Could you check a few things on this drawing? It's one solid part, dimensions in mm from its lowest x, y, z. Coordinates: 2 decimals unless noted, no trailing zeros. Order: outer loops, then holes, each group sorted by start corner. A loop starts at its lowest first (then second) coordinate and runs counter-clockwise, first axis right, second up.
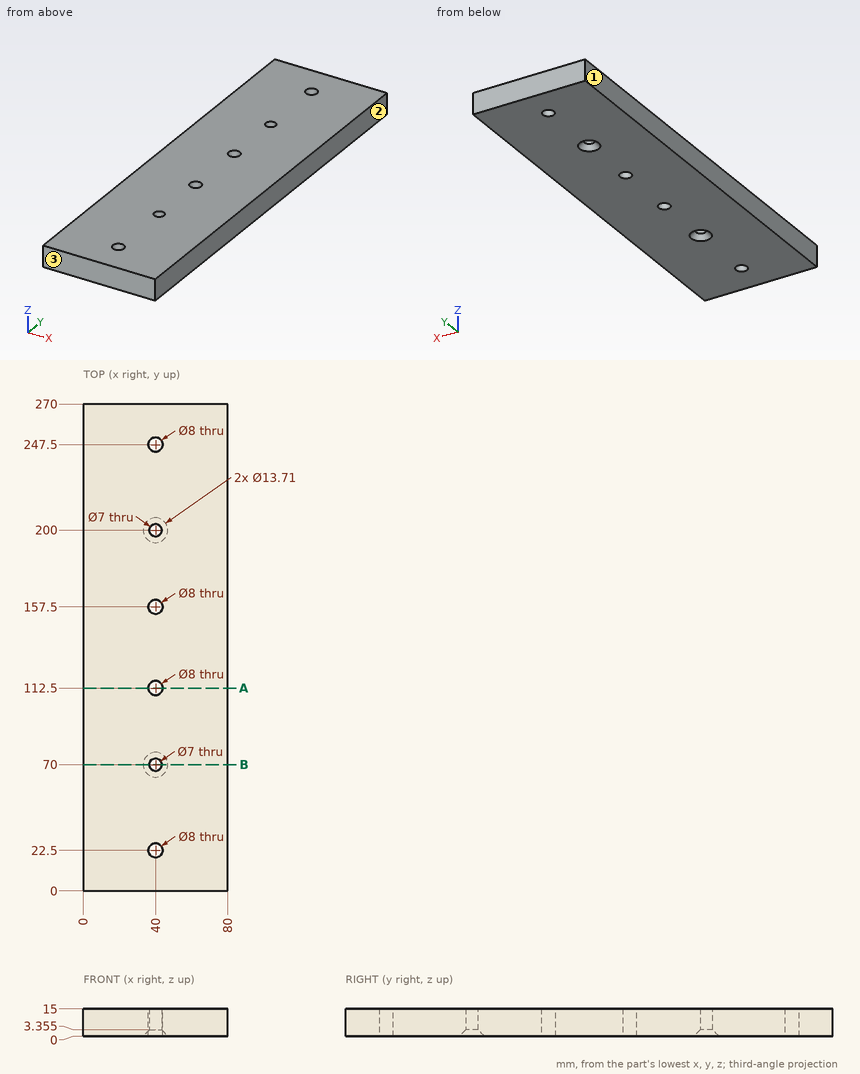
1. Imagine slicing it at A-A on y = 112.5. Please give me the cut outline in (x, z).
Completed:
outline: (0, 0) - (36, 0) - (36, 15) - (0, 15) - close; (44, 0) - (80, 0) - (80, 15) - (44, 15) - close
2. Please list where these lines run through material, in increasing order: probe 1 along X at (y, z) = (70, 10.5); probe 2 along X at (y, z) = (112.5, 4.5).
Completed:
probe 1: x = 0 to 36.5, 43.5 to 80
probe 2: x = 0 to 36, 44 to 80
3. Thinking about a two-plate mould opening in X: for the marked faces 1, 2 and 3, which applies, pulls with the +X half, pulls with the -X half, needs draft (parallel to the pull), parting line crosses it, or undercut?
Completed:
face 1: pulls with the -X half
face 2: pulls with the +X half
face 3: needs draft
4. Imagine slicing it at B-B on y = 70. Please give me the cut outline in (x, z) (3 decimals).
Completed:
outline: (0, 0) - (33.145, 0) - (36.5, 3.355) - (36.5, 15) - (0, 15) - close; (43.5, 3.355) - (46.855, 0) - (80, 0) - (80, 15) - (43.5, 15) - close
5. I'm going to push a flat-ended pin straight in: pin 1 (6.5 mm diameter, centred on x = 40, y = 112.5, fed in from -Z). Where does the tip first touch, or does it pass through?
Completed:
pin 1: passes through
